from build123d import *

# Parameters (mm, degrees)
SKETCH1_R       = 215
SKETCH1_R_2     = 50
LID_DEPTH       = 6
SKETCH2_R       = 2.75
ROD_HOLES_DEPTH = 6


with BuildPart() as part:
    # Sketch1 → Lid (new body)
    with BuildSketch(Plane.XY):
        Circle(SKETCH1_R)
        Circle(SKETCH1_R_2, mode=Mode.SUBTRACT)
    extrude(amount=LID_DEPTH)

    # Sketch2 → Rod_holes (cut)
    with BuildSketch(Plane.XY):
        with Locations((198.770811906, 64.584551824)):
            Circle(SKETCH2_R)
        with Locations((0, 209)):
            Circle(SKETCH2_R)
        with Locations((-198.770811906, 64.584551824)):
            Circle(SKETCH2_R)
        with Locations((-122.847117729, -169.084551824)):
            Circle(SKETCH2_R)
        with Locations((122.847117729, -169.084551824)):
            Circle(SKETCH2_R)
    extrude(amount=ROD_HOLES_DEPTH, mode=Mode.SUBTRACT)


solid = part.part
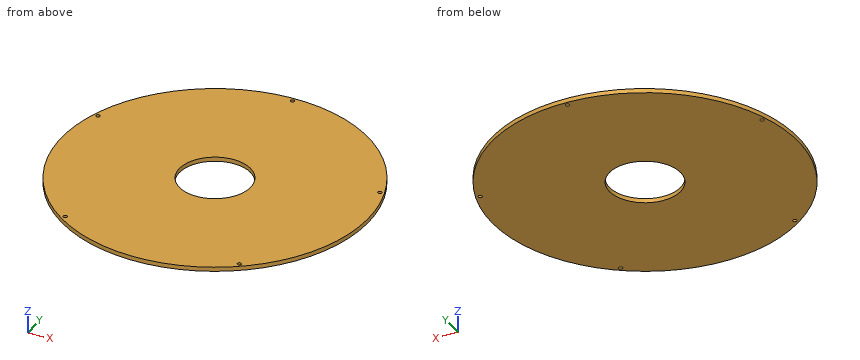
Can you work these out from the model? Positions are in its coordinate system, mm. Coordinates: 2 decimals unless noted, no trailing zeros. Order: outer loops, then holes, each group sorted by start corner. A loop starts at its lowest first (then second) coordinate and runs counter-clockwise, first axis right, second up. Notation, with made-up numbers: M -5,-40 L 4,-40 A25 cw 4,-22 Z; hole C 16.5,21.5 d2. An arc over 180 degrees is marked long. Write item = value, one per line.
(1) Suppose I cut it at B-B on x = -27. Please give me the cut outline in (y, z).
Results are:
outline = M -213.3,0 L -42.08,0 L -42.08,6 L -213.3,6 Z; M 42.08,0 L 213.3,0 L 213.3,6 L 42.08,6 Z
(2) Suppose I cut it at A-A on y = 0. Please give me the cut outline in (x, z), plus the area to 3 significant figures.
Results are:
outline = M -215,0 L -50,0 L -50,6 L -215,6 Z; M 50,0 L 215,0 L 215,6 L 50,6 Z
area = 1,980 mm2
(3) I need wall thicknesses on line 1 along Y through (x, z) = (0, 2.5); line 2 along Y through (x, z) = (-10.5, 3.2); line 3 along X through (y, z) = (45, 1.95). Which ranges of each line are inside material? Lowest first, please. Write a range as [from, to].
Results are:
line_1 = [-215, -50], [50, 206.25], [211.75, 215]
line_2 = [-214.74, -48.89], [48.89, 214.74]
line_3 = [-210.24, -21.79], [21.79, 210.24]
(4) Suppose I cut it at C-C on z = 2.1. Please give me the cut outline in (x, y), plus the area to 3 significant figures.
Results are:
outline = C 0,0 d430; hole C -198.77,64.58 d5.5; hole C -122.85,-169.08 d5.5; hole C 0,0 d100; hole C 0,209 d5.5; hole C 122.85,-169.08 d5.5; hole C 198.77,64.58 d5.5
area = 137,000 mm2
(5) For pin 1 Ø9 at (x, y) = (-198.77, 64.58) entering from +Z; pin 2 Ø1 at (y, z) = (-121.5, 4.5) entering from -X; pin 3 Ø1 at (y, z) = (19.5, 3.5) entering from +X; pin 4 Ø2 at (x, z) = (88, 4) entering from -Y, each with a flat end and sliding along its axis, tell me the tip position at first contact or that it passes through.
Results are:
pin_1 = 6
pin_2 = -177.72
pin_3 = 214.16
pin_4 = -196.61
(6) Suppose I cut it at D-D on x = -79. Please give me the cut outline in (y, z).
Results are:
outline = M -199.96,0 L 199.96,0 L 199.96,6 L -199.96,6 Z
